```python
from build123d import *

# Parameters (mm, degrees)
CROSSHEAD_START = 54
SKETCH1_W       = 4.5
SKETCH1_H       = 4
CROSSHEAD_DEPTH = 25
ROD_SLOT_START  = 63.24
SKETCH2_W       = 2.2
SKETCH2_H       = 1.6
ROD_SLOT_DEPTH  = 6.2


with BuildPart() as part:
    # Sketch1 → crosshead (new body)
    with BuildSketch(Plane(origin=(0, 0, 0), x_dir=(0, 0, -1), z_dir=(1, 0, 0)).offset(CROSSHEAD_START)):
        with Locations((-36.75, 178)):
            Rectangle(SKETCH1_W, SKETCH1_H)
    extrude(amount=CROSSHEAD_DEPTH)


with BuildPart() as body_2:
    # Sketch2 → rod_slot (new body)
    with BuildSketch(Plane(origin=(0, 0, 0), x_dir=(0, 0, -1), z_dir=(1, 0, 0)).offset(ROD_SLOT_START)):
        with Locations((-36.5, 176.7)):
            Rectangle(SKETCH2_W, SKETCH2_H)
    extrude(amount=ROD_SLOT_DEPTH)


with BuildPart() as part_1:
    add(part.part)

    # Combine1: cut body 2
    add(body_2.part, mode=Mode.SUBTRACT)


solid = part_1.part
```
CAD build for the part. Positions are in the model's coordinates, mm. A direction names the side the tool comes from. Coordinates: 2 decimals unless noted, no trailing zeros. Order: outer loops, then holes, each group sorted by start corner. A loop starts at its lowest first (then second) coordinate and runs counter-clockwise, first axis right, second up. Notation, with made-up numbers: M 14,27 L 46,27 A14 ccw 46,44 Z; hole C 54.25,-29.5 d8. An arc over 180 degrees is marked long. Write each question's results on one line, items separated by ' | '. Start each with the question number.
Q1. Drill centre lines: probe 1 along X at (y, z) = (177.05, 36.85); probe 2 along Z at (x, y) = (68.25, 176.8); probe 3 along Y at (x, z) = (65.5, 36.25). Where is each one in solid material? Low to high. Write a range as from..to.
Q2. Cut at B-B (x = 63.5). List the corners of the cut face in (y, z), then the cut area to 3 significant figures.
Q3. Pull direction X, two halves, no side cores. Call faces 3 (the flat face through (63.24, 177, 37)), 4 (the flat face through (66, 177.5, 37)), 5 (the flat face through (54, 178, 37)), 6 (the flat face through (66, 176, 38)): +X half, -X half, draft (parallel to the pull), parting line (faces both ways), or undercut.
Q4. Which spindle directions (+Z, -Z, +X, -X, +Y, -Y) get a long thin tool onto all of the face, cutting with end or side? Do faces 1 (the flat face through (66, 180, 37)), 2 (the flat face through (66, 177, 37.6)). Say none if no direction does.
Q5. Cut at A-A (y = 177). List the corners of the cut face in (x, z).
Q6. Cut at C-C (z = 37.2). List the corners of the cut face in (x, y), then the cut area to 3 significant figures.
Q7. Flat gauge pin, fed straight in: P1, Ø1.1, axis at x = 66.5, z = 36.5, coming from the -Y side. Where does the tip first touch, or does it go through?
Found:
1) probe 1: 54..63.24, 69.44..79 | probe 2: 34.5..35.4, 37.6..39 | probe 3: 177.5..180
2) outline: M 176,34.5 L 180,34.5 L 180,39 L 176,39 L 176,37.6 L 177.5,37.6 L 177.5,35.4 L 176,35.4 Z | area: 14.7 mm²
3) face 3: undercut | face 4: undercut | face 5: -X half | face 6: draft
4) face 1: +Z, -Z, +X, -X, +Y | face 2: -Y
5) outline: M 54,34.5 L 79,34.5 L 79,39 L 54,39 Z; hole M 63.24,35.4 L 69.44,35.4 L 69.44,37.6 L 63.24,37.6 Z
6) outline: M 54,176 L 63.24,176 L 63.24,177.5 L 69.44,177.5 L 69.44,176 L 79,176 L 79,180 L 54,180 Z | area: 90.7 mm²
7) P1: y = 177.5
